The listing builds one solid part. Answer for the finished solid, in the listing's coordinates (mm). A direction names the side the tool comes from. Give positions to 0.01 mm unless a question says otherwise; leave off trailing zeros. Loops run counter-clockwise (first coordinate to the right, second up) from the corner with the lowest first, then second, coordinate; pieces in that order, holes last. Notation, with made-up numbers: (60, 77.25) - (72, 77.25) arc R9 ccw to (72, 82.25) - close; hole circle Ø8 at (84.25, 48). An arc over 180 degrees is marked (long way). Write each question's results on one line, items separated by ' | '.
from build123d import *

# Parameters (mm, degrees)
CROQUIS4_R              = 95.5
CROQUIS4_R_2            = 79
CORTAR_EXTRUIR1_START   = -79
CROQUIS6_R              = 85
CROQUIS6_R_2            = 79
CORTAR_EXTRUIR1_DEPTH   = 79
CROQUIS7_R              = 85
CROQUIS7_R_2            = 79
CORTAR_EXTRUIR2_DEPTH   = 79
CROQUIS8_R              = 95.5
CORTAR_EXTRUIR3_DEPTH   = 79
CROQUIS10_R             = 4
SALIENTE_EXTRUIR3_DEPTH = 10
CROQUIS11_R             = 95.5
CORTAR_EXTRUIR4_DEPTH   = 351.943371662
CROQUIS12_R             = 4
SALIENTE_EXTRUIR4_DEPTH = 10


with BuildPart() as part:
    # Barrer5: sweep along a path in Croquis3
    with BuildLine(Plane.XY) as barrer5_path:
        Line((0, 0), (0, 79))
        ThreePointArc((0, 79), (29.435768491, 150.064231509), (100.5, 179.5))
        Line((100.5, 179.5), (179.5, 179.5))
    # Croquis4 → Barrer5 (sweep)
    with BuildSketch(Plane(origin=(0, 0, 0), x_dir=(1, 0, 0), z_dir=(0, 1, 0))):
        Circle(CROQUIS4_R)
        Circle(CROQUIS4_R_2, mode=Mode.SUBTRACT)
    sweep(path=barrer5_path.line)

    # Croquis6 → Cortar-Extruir1 (cut)
    with BuildSketch(Plane.XZ.offset(CORTAR_EXTRUIR1_START)):
        with Locations(Location((0, 0, 0), (0, 0, 270))):
            Circle(CROQUIS6_R)
        Circle(CROQUIS6_R_2, mode=Mode.SUBTRACT)
    extrude(amount=CORTAR_EXTRUIR1_DEPTH, mode=Mode.SUBTRACT)

    # Croquis7 → Cortar-Extruir2 (cut)
    with BuildSketch(Plane(origin=(179.5, 0, 0), x_dir=(0, 0, -1), z_dir=(1, 0, 0))):
        with Locations(Location((0, 179.5, 0), (0, 0, 90))):
            Circle(CROQUIS7_R)
        with Locations((0, 179.5)):
            Circle(CROQUIS7_R_2, mode=Mode.SUBTRACT)
    extrude(amount=-CORTAR_EXTRUIR2_DEPTH, mode=Mode.SUBTRACT)

    # Croquis8 → Cortar-Extruir3 (cut)
    with BuildSketch(Plane.XZ.offset(-79)):
        Circle(CROQUIS8_R)
    extrude(amount=CORTAR_EXTRUIR3_DEPTH, mode=Mode.SUBTRACT)

    # Croquis10 → Saliente-Extruir3 (add)
    with BuildSketch(Plane.XZ.offset(-79)):
        with Locations(Location((0, 89.75, 0), (0, 0, 270))):
            Circle(CROQUIS10_R)
        with Locations(Location((70.169375552, 55.958209717, 0), (0, 0, 270))):
            Circle(CROQUIS10_R)
        with Locations(Location((87.499780118, -19.971253823, 0), (0, 0, 270))):
            Circle(CROQUIS10_R)
        with Locations(Location((38.941065586, -80.861955894, 0), (0, 0, 270))):
            Circle(CROQUIS10_R)
        with Locations(Location((-38.941065586, -80.861955894, 0), (0, 0, 270))):
            Circle(CROQUIS10_R)
        with Locations(Location((-87.499780118, -19.971253823, 0), (0, 0, 270))):
            Circle(CROQUIS10_R)
        with Locations(Location((-70.169375552, 55.958209717, 0), (0, 0, 270))):
            Circle(CROQUIS10_R)
    extrude(amount=SALIENTE_EXTRUIR3_DEPTH)

    # Croquis11 → Cortar-Extruir4 (cut, through all)
    with BuildSketch(Plane(origin=(100.5, 0, 0), x_dir=(0, 0, -1), z_dir=(1, 0, 0))):
        with Locations((0, 179.5)):
            Circle(CROQUIS11_R)
    extrude(amount=CORTAR_EXTRUIR4_DEPTH, mode=Mode.SUBTRACT)

    # Croquis12 → Saliente-Extruir4 (add)
    with BuildSketch(Plane(origin=(100.5, 0, 0), x_dir=(0, 0, -1), z_dir=(1, 0, 0))):
        with Locations(Location((0, 269.25, 0), (0, 0, 90))):
            Circle(CROQUIS12_R)
        with Locations(Location((70.169375552, 235.458209717, 0), (0, 0, 90))):
            Circle(CROQUIS12_R)
        with Locations(Location((87.499780118, 159.528746177, 0), (0, 0, 90))):
            Circle(CROQUIS12_R)
        with Locations(Location((38.941065586, 98.638044106, 0), (0, 0, 90))):
            Circle(CROQUIS12_R)
        with Locations(Location((-38.941065586, 98.638044106, 0), (0, 0, 90))):
            Circle(CROQUIS12_R)
        with Locations(Location((-87.499780118, 159.528746177, 0), (0, 0, 90))):
            Circle(CROQUIS12_R)
        with Locations(Location((-70.169375552, 235.458209717, 0), (0, 0, 90))):
            Circle(CROQUIS12_R)
    extrude(amount=SALIENTE_EXTRUIR4_DEPTH)


solid = part.part
Item 1: For faces 1 (the face through (105.43, 234.591, 66.264)), 2 (the face through (88, 69, -20)), 3 (the face through (-71, 79, 36)), determine the directions among +Z, -Z, +X, -X, +Y, -Y from which every point of the face is accessible in a straight line to the end or side of a thin tool.
Values found:
face 1: +X | face 2: +Z, -Z, +X, -X, -Y | face 3: -Y
Item 2: Find the intervals of material crossed by line 1 along Z through (x, y) = (63, 174); line 2 along Z through (x, y) = (98.5, 164); line 3 along Y through (x, z) = (73, 45.5), in increasing order. Write a range as [from, to].
Values found:
line 1: z = [-95.49, -78.98], [78.98, 95.49] | line 2: z = [-94.24, -77.47], [77.47, 94.24] | line 3: y = [79, 102.11], [241.77, 261.4]
Item 3: A cutting plane is placed at A-A, the plane z = 0. Determine the outline of the cut face in (x, y).
Values found:
outline: (-95.5, 79) - (-79, 79) arc R179.5 cw to (100.5, 258.5) - (100.5, 265.25) - (110.5, 265.25) - (110.5, 273.25) - (100.5, 273.25) - (100.5, 275) arc R196 ccw to start; (79, 79) - (95.5, 79) arc R5 cw to (100.5, 84) - (100.5, 100.5) arc R21.5 ccw to start
Item 4: Flat-ended cylindrical pins translate along their axes: P1, Ø2, axis at y = 167, z = -60.5, coming from the +X side; P2, Ø10, axis at y = 110, z = -24.5, coming from the -X side; P3, Ø12, axis at x = 44.5, z = -66, coming from the +Y side. Find the tip coordinate at first contact, or state that the pin passes through.
Values found:
P1: stops at x = -20.92 | P2: stops at x = -91.24 | P3: stops at y = 244.96
Item 5: For a pull along Z with two mould halves and no side action, classify faces 4 (the face through (41.64, 74.07, -77.91)), 5 (the face through (110.5, 269, 0)), 6 (the face through (105.43, 234.591, -74.074)) as released by +Z, released by -Z, zero draft, split by the parting line, or undercut.
Values found:
face 4: split by the parting line | face 5: zero draft | face 6: undercut
